from build123d import *
from OCP.BRepFilletAPI import BRepFilletAPI_MakeChamfer

# Parameters (mm, degrees)
SKETCH1_W           = 30.5
SKETCH1_H           = 30.5
BOSS_EXTRUDE1_DEPTH = 10
SKETCH2_W           = 30.5
SKETCH2_H           = 30.5
BOSS_EXTRUDE2_DEPTH = 30
CHAMFER1_SIZE       = 10
CHAMFER1_SIZE2      = 11.831007916
SKETCH3_R           = 2
CUT_EXTRUDE1_DEPTH  = 94.224303623
SKETCH4_R           = 2
CUT_EXTRUDE2_DEPTH  = 120.721978802
SKETCH5_R           = 2
CUT_EXTRUDE3_DEPTH  = 30
SKETCH6_R           = 2
CUT_EXTRUDE4_DEPTH  = 122.429059078
CHAMFER3_SIZE       = 2


with BuildPart() as part:
    # Sketch1 → Boss-Extrude1 (new body)
    with BuildSketch(Plane.XY):
        Polygon((-25, -60.25), (-25, -13.014176264), (-64.503552507, 14.646508987), (-35.824730689, 55.604111202), (0, 30.519364719), (35.824730689, 55.604111202), (64.503552507, 14.646508987), (25, -13.014176264), (25, -60.25), align=None)
        Rectangle(SKETCH1_W, SKETCH1_H, mode=Mode.SUBTRACT)
    extrude(amount=BOSS_EXTRUDE1_DEPTH)

    # Sketch2 → Boss-Extrude2 (add)
    with BuildSketch(Plane.XY.offset(10)):
        Polygon((-58.767788143, 22.83802943), (-34.193226815, 5.63073634), (-16.985933724, 30.205297668), (-41.560495053, 47.412590759), (-35.824730689, 55.604111202), (0, 30.519364719), (35.824730689, 55.604111202), (41.560495053, 47.412590759), (16.985933724, 30.205297668), (34.193226815, 5.63073634), (58.767788143, 22.83802943), (64.503552507, 14.646508987), (25, -13.014176264), (25, -60.25), (15, -60.25), (15, -30.25), (-15, -30.25), (-15, -60.25), (-25, -60.25), (-25, -13.014176264), (-64.503552507, 14.646508987), align=None)
        Rectangle(SKETCH2_W, SKETCH2_H, mode=Mode.SUBTRACT)
    extrude(amount=BOSS_EXTRUDE2_DEPTH)

    # Chamfer1: one chamfer whose edges measure the first distance from different faces: ONE call of the kernel's chamfer builder (chamfer() names one face for all edges)
    chamfer1_edges_1 = [part.edges().sort_by_distance(p)[0] for p in [
        (-25, -13.014176264, 20),
    ]]
    chamfer1_side_1 = [part.faces().sort_by_distance(p)[0] for p in [
        (-25, -36.632088132, 20),
    ]]
    chamfer1_edges_2 = [part.edges().sort_by_distance(p)[0] for p in [
        (25, -13.014176264, 20),
    ]]
    chamfer1_side_2 = [part.faces().sort_by_distance(p)[0] for p in [
        (25, -36.632088132, 20),
    ]]
    chamfer1 = BRepFilletAPI_MakeChamfer(part.part.solid().wrapped)
    for e in chamfer1_edges_1:
        chamfer1.Add(CHAMFER1_SIZE, CHAMFER1_SIZE2, e.wrapped, chamfer1_side_1[0].wrapped)  # the first distance lies on this face
    for e in chamfer1_edges_2:
        chamfer1.Add(CHAMFER1_SIZE, CHAMFER1_SIZE2, e.wrapped, chamfer1_side_2[0].wrapped)  # the first distance lies on this face
    add(Compound.cast(chamfer1.Shape()), mode=Mode.REPLACE)

    # Chamfer2
    # the kernel refuses this chamfer: 10 mm, written as the material it adds along each edge
    with BuildSketch(Plane(origin=(0, 30.519364719, 40), x_dir=(0.8366959699781049, 0.5476676490558834, 0), z_dir=(0, 0, -1))) as chamfer2_piece_1:
        with BuildLine():
            Line((7.333326063, 0), (-2.934212568, -6.720719288))
            Line((-2.934212568, -6.720719288), (-3.119919002, -6.646468897))
            ThreePointArc((-3.119919002, -6.646468897), (-1.546295883, -3.328697528), (-0.185706433, 0.074250391))
            Line((-0.185706433, 0.074250391), (0.006257204, 0.199902095))
            ThreePointArc((0.006257204, 0.199902095), (3.669331251, 0.085242964), (7.339583267, 0.199902095))
            Line((7.339583267, 0.199902095), (7.333326063, 0))
        make_face()
    extrude(amount=40)

    # Sketch3 → Cut-Extrude1 (cut, through all)
    with BuildSketch(Plane.XY.offset(10)):
        with Locations((37.876860934, 26.521663549)):
            Circle(SKETCH3_R)
        with Locations((0, -45.25)):
            Circle(SKETCH3_R)
        with Locations((-37.876860934, 26.521663549)):
            Circle(SKETCH3_R)
    extrude(amount=-CUT_EXTRUDE1_DEPTH, mode=Mode.SUBTRACT)

    # Sketch4 → Cut-Extrude2 (cut, through all)
    with BuildSketch(Plane(origin=(-14.339410909, 20.478801107, 0), x_dir=(0.819152044288991, 0.5735764363510474, 0), z_dir=(-0.5735764363510474, 0.819152044288991, 0))):
        with Locations(Location((46.23910933, -25, 0), (0, 0, 180))):
            Circle(SKETCH4_R)
    cut_extrude2 = extrude(amount=-CUT_EXTRUDE2_DEPTH, mode=Mode.SUBTRACT)

    # Sketch5 → Cut-Extrude3 (cut)
    with BuildSketch(Plane(origin=(25, 0, 0), x_dir=(0, 0, -1), z_dir=(1, 0, 0))):
        with Locations(Location((-25, -45.25, 0), (0, 0, 90))):
            Circle(SKETCH5_R)
    cut_extrude3 = extrude(amount=-CUT_EXTRUDE3_DEPTH, mode=Mode.SUBTRACT)

    # Mirror1: Cut-Extrude2, Cut-Extrude3 across plane
    add(cut_extrude2.mirror(Plane(origin=(0, 0, 0), x_dir=(0, 0, 1), z_dir=(1, 0, 0))), mode=Mode.SUBTRACT)
    add(cut_extrude3.mirror(Plane(origin=(0, 0, 0), x_dir=(0, 0, 1), z_dir=(1, 0, 0))), mode=Mode.SUBTRACT)

    # Sketch6 → Cut-Extrude4 (cut, through all)
    with BuildSketch(Plane(origin=(0, 34.535590164, 0), x_dir=(1, 0, 0), z_dir=(0, 1, 0))):
        with Locations(Location((0, -20, 0), (0, 0, 270))):
            Circle(SKETCH6_R)
    extrude(amount=-CUT_EXTRUDE4_DEPTH, mode=Mode.SUBTRACT)

    # Chamfer3
    chamfer3_edges = [part.edges().sort_by_distance(p)[0] for p in [
        (35.876860934, 26.521663549, 0),
        (-2, -45.25, 0),
        (-39.876860934, 26.521663549, 0),
        (53.854575931, 7.190015315, 25),
        (25.175754113, 48.147617529, 25),
        (25, -47.25, 25),
        (-25.175754113, 48.147617529, 25),
        (-53.854575931, 7.190015315, 25),
        (-25, -47.25, 25),
        (0, -30.25, 18),
        (0, 34.535590164, 18),
    ]]
    chamfer(chamfer3_edges, length=CHAMFER3_SIZE)


solid = part.part
Work out the finished part from the listing and answer in its coordinate system (mm). A direction names the side the tool comes from. Round coordinates to 2 decimals unless told otherwise and drop trailing zeros. Loops run counter-clockwise (first coordinate to the right, second up) from the corner with the lowest first, then second, coordinate; pieces in that order, holes last. Notation, with made-up numbers: (85.5, 16) - (113.5, 16) arc R19 cw to (113.5, 34) - close; hole circle Ø3 at (-10, 66). An arc over 180 degrees is marked (long way). Use one line per item in the form item = value. Start each with the question number.
(1) Find section D-D on y = 21. Determine the outline of the cut face in (x, z), and give its area (3 significant figures).
(2) Determine the mould class of faces 1 (the face through (50.04, 11.91, 23.78)), 2 (the face through (15.25, 0, 20)), 3 (the face through (34, 27, 10)) for opening direction Z: +Z half, -Z half, draft (parallel to the pull), parting line (faces both ways), or undercut.
(3) Which of the six approach directions +Z, -Z, +X, -X, +Y, -Y give full straight-line access (tool end or side, diameter ignored) to faces 4 (the face through (-25.71, 17.746, 24.79)), 5 (the face through (-20.991, 45.217, 19.72)), 6 (the face through (-25, -42, 20))?
(4) Find section B-B on y = -45.25. Determine the outline of the cut face in (x, z).
(5) Consider line 1 (Y direction, x = 0, z = 6.75); line 2 (X direction, y = -54.5, z = 22); line 3 (Y direction, x = 1, z = 25.5). Determine where each line is inside the solid, lowest interval first.
(6) Find section A-A on x = 0. Determine the outline of the cut face in (y, z), and give its area (3 significant figures).
(7) Flat-ended cylindrical pins translate along their axes: P1, Ø1.5, axis at y = 3, z = 7, coming from the +X side; P2, Ø21, axis at x = -30, y = 17, coming from the +Z side; P3, Ø12, axis at x = -7.5, z = 15.5, coming from the +Y side; P4, Ø6, axis at x = -48, z = 30.5, coming from the -Y side. Find the tip coordinate at first contact, or state that the pin passes through.
(8) Find section C-C on z = 14. Determine the outline of the cut face in (x, y), and give its area (3 significant figures).
Answer list:
q1.outline = (-60.05, 0) - (60.05, 0) - (60.05, 40) - (56.14, 40) - (56.14, 10) - (23.43, 10) - (23.43, 40) - (-23.43, 40) - (-23.43, 10) - (-56.14, 10) - (-56.14, 40) - (-60.05, 40) - close; hole circle Ø4 at (0, 20)
q1.area = 2,830 mm^2
q2.face_1 = undercut
q2.face_2 = draft
q2.face_3 = +Z half
q3.face_4 = +Z
q3.face_5 = +Z, -Z, +Y
q3.face_6 = +Z, -Z, -X, -Y
q4.outline = (-25, 0) - (-4, 0) - (-2, 2) - (-2, 10) - (-15, 10) - (-15, 23) - (-23, 23) - (-25, 21) - close; (-25, 29) - (-23, 27) - (-15, 27) - (-15, 40) - (-25, 40) - close; (2, 2) - (4, 0) - (25, 0) - (25, 21) - (23, 23) - (15, 23) - (15, 10) - (2, 10) - close; (15, 27) - (23, 27) - (25, 29) - (25, 40) - (15, 40) - close
q5.line_1 = -60.25 to -47.25, -43.25 to -15.25, 15.25 to 34.54
q5.line_2 = -25 to -15, 15 to 25
q5.line_3 = -30.25 to -15.25, 15.25 to 34.54
q6.outline = (-60.25, 0) - (-49.25, 0) - (-47.25, 2) - (-47.25, 10) - (-60.25, 10) - close; (-43.25, 2) - (-41.25, 0) - (-15.25, 0) - (-15.25, 18) - (-28.25, 18) - (-30.25, 16) - (-30.25, 10) - (-43.25, 10) - close; (-30.25, 24) - (-28.25, 22) - (-15.25, 22) - (-15.25, 40) - (-30.25, 40) - close; (15.25, 0) - (34.54, 0) - (34.54, 16) - (32.54, 18) - (15.25, 18) - close; (15.25, 22) - (32.54, 22) - (34.54, 24) - (34.54, 40) - (15.25, 40) - close
q6.area = 1,480 mm^2
q7.P1 = 48.94
q7.P2 = 40
q7.P3 = 39.97
q7.P4 = 0.99
q8.outline = (-64.5, 14.65) - (-34.69, -6.23) - (-25, -23.01) - (-25, -60.25) - (-15, -60.25) - (-15, -30.25) - (15, -30.25) - (15, -60.25) - (25, -60.25) - (25, -23.01) - (34.69, -6.23) - (64.5, 14.65) - (58.77, 22.84) - (34.19, 5.63) - (16.99, 30.21) - (41.56, 47.41) - (35.82, 55.6) - (5.74, 34.54) - (-5.74, 34.54) - (-35.82, 55.6) - (-41.56, 47.41) - (-16.99, 30.21) - (-34.19, 5.63) - (-58.77, 22.84) - close; hole (-15.25, -15.25) - (15.25, -15.25) - (15.25, 15.25) - (-15.25, 15.25) - close
q8.area = 4,540 mm^2
